Study the drawing (mm; zero at the part's minimum x, y, z) and answer. A direction names the side the tool comes from. Round coordinates to 2 decimals unless told otherwise and drop trailing zeros. Order: outer loops, then holes, each group sorted by start corner. A loop starts at its lowest first (then second) coordinate and runs counter-clockwise, first axis right, second up. Notation, with made-up numbers: (65, 81.25) - (114, 81.25) arc R20 ccw to (114, 107.25) - close; hole circle Ø4 at (53, -39.5). An arc over 180 degrees is marked (long way). Use one line per item in the form item = value. Start each with the question number.
Q1. Which of the six approach directions +Z, -Z, +X, -X, +Y, -Y give full straight-line access (tool end or side, diameter ignored) to the marked faces 1 and 2?
Q2. The part is cut by section A-A on y = 35. Determine the outline of the cut face in (x, z).
Q3. The part is cut by section B-B on x = 16.5. Determine the outline of the cut face in (y, z), plus the area to 3 significant figures.
Q4. Given P1, Ø1.5, axis at x = 20, z = 15, coming from the +Y side; P2, Ø6, axis at x = 37, y = 12, coming from the -Z side; P3, Ø12, axis at y = 40, z = 12, coming from the -X side, each flat-ended and moving along its own axis, determine where each tip first touches the part or whether it passes through.
Q5. The part is cut by section C-C on z = 19.75. Determine the outline of the cut face in (x, y), plus the area to 3 significant figures.
Q6. The part is cut by section D-D on y = 22. Determine the outline of the cut face in (x, z).
Q7. Find the intervals of material crossed by line 1 (Z direction, x = 20.5, y = 38); line 2 (Y direction, x = 39, z = 5.75), in increasing order. Write a range as [from, to].
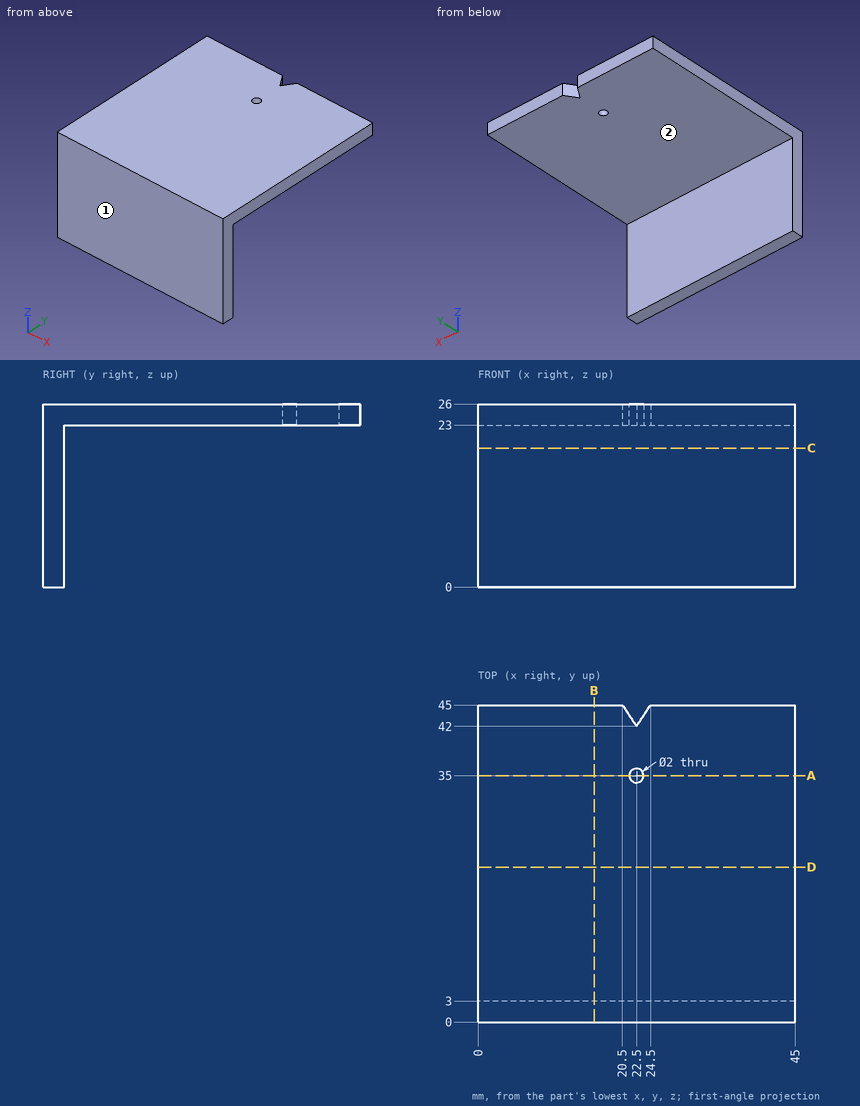
Found:
q1.face_1 = +Z, -Z, +X, -X, -Y
q1.face_2 = -Z, +X, -X, +Y
q2.outline = (0, 23) - (21.5, 23) - (21.5, 26) - (0, 26) - close; (23.5, 23) - (45, 23) - (45, 26) - (23.5, 26) - close
q3.outline = (0, 0) - (3, 0) - (3, 23) - (45, 23) - (45, 26) - (0, 26) - close
q3.area = 204 mm²
q4.P1 = 3
q4.P2 = 23
q4.P3 = through
q5.outline = (0, 0) - (45, 0) - (45, 3) - (0, 3) - close
q5.area = 135 mm²
q6.outline = (0, 23) - (45, 23) - (45, 26) - (0, 26) - close
q7.line_1 = [23, 26]
q7.line_2 = [0, 3]
